Geometry: final body of the model. Coordinates: model frame, mm. A direction names the side the tool comes from. Give positions to 0.01 mm unless a question says otherwise; leave off trailing zeros. Write each loop counter-clockwise with the first axis right and the second up, starting at its lowest first coordinate (ties: lowest second). Pieces come first, ordered by that corner, then holes. Notation, with made-up numbers: M 14,8.25 L 61,8.25 A19 ccw 61,37.25 Z; hole C 78.25,0.25 d10. An arc over 180 degrees is marked long. Answer as a JSON object with one key per item and string values.
from build123d import *

# Parameters (mm, degrees)
F0_R     = 17.5
F1_DEPTH = 5
F2_R     = 15.5
F3_DEPTH = 3
F4_R     = 3.5
F4_R_2   = 1.5
F5_DEPTH = 6
F7_DEPTH = 1
F8_DEPTH = 2


with BuildPart() as f1:
    # F0 (on Top) → F1 (new body)
    with BuildSketch(Plane.XY):
        Circle(F0_R)
    extrude(amount=F1_DEPTH)

    # F2 (on face) → F3 (cut)
    with BuildSketch(Plane.XY.offset(5)):
        Circle(F2_R)
    extrude(amount=-F3_DEPTH, mode=Mode.SUBTRACT)

    # F4 (on face) → F5 (join)
    with BuildSketch(Plane.XY.offset(2)):
        Circle(F4_R)
        Circle(F4_R_2, mode=Mode.SUBTRACT)
    extrude(amount=F5_DEPTH)

    # F6 (on face) → F7 (cut)
    with BuildSketch(Plane(origin=(0, 0, 0), x_dir=(1, 0, 0), z_dir=(0, 0, -1))):
        Polygon((-3.9243327608, 0.1564746204), (-3.3940706843, 1.1028004157), (-3.2668253693, 2.1800742948), (-12.161596097, 3.9515421095), align=None)
        Polygon((1.0638693073, 3.7806155611), (0, 12.7874588824), (-1.0638693073, 3.7806155611), (0, 3.5687371109), align=None)
        Polygon((3.2668253693, 2.1800742948), (3.3940706843, 1.1028004157), (3.9243327608, 0.1564746204), (12.161596097, 3.9515421095), align=None)
        Polygon((3.0828784209, -2.4332555489), (2.0976510431, -2.8871689712), (1.361501722, -3.6839089274), (7.5162797454, -10.3452715508), align=None)
        Polygon((-1.361501722, -3.6839089274), (-2.0976510431, -2.8871689712), (-3.0828784209, -2.4332555489), (-7.5162797454, -10.3452715508), align=None)
    extrude(amount=-F7_DEPTH, mode=Mode.SUBTRACT)

    # F6 (on face) → F8 (cut)
    with BuildSketch(Plane(origin=(0, 0, 0), x_dir=(1, 0, 0), z_dir=(0, 0, -1))):
        with BuildLine():
            Line((7.6763518896, -13.4656459803), (0, -5.1574724983))
            Line((0, -5.1574724983), (-7.6763518896, -13.4656459803))
            ThreePointArc((-7.6763518896, -13.4656459803), (0, -15.5), (7.6763518896, -13.4656459803))
        make_face()
        with BuildLine():
            Line((-10.434467167, -11.4617579341), (-4.9050478272, -1.59374665))
            Line((-4.9050478272, -1.59374665), (-15.1787135444, 3.1395310378))
            ThreePointArc((-15.1787135444, 3.1395310378), (-14.7413760026, -4.7897634128), (-10.434467167, -11.4617579341))
        make_face()
        with BuildLine():
            Line((1.7046089863, 15.4059828704), (3.0314862736, 4.1724828992))
            Line((3.0314862736, 4.1724828992), (14.1252072533, 6.3818900062))
            ThreePointArc((14.1252072533, 6.3818900062), (9.1106714105, 12.5397634128), (1.7046089863, 15.4059828704))
        make_face()
        with BuildLine():
            Line((15.1787135444, 3.1395310378), (4.9050478272, -1.59374665))
            Line((4.9050478272, -1.59374665), (10.434467167, -11.4617579341))
            ThreePointArc((10.434467167, -11.4617579341), (14.1771689891, -6.2656108605), (15.5, 0))
            ThreePointArc((15.5, 0), (15.4194691857, 1.5779638877), (15.1787135444, 3.1395310378))
        make_face()
        with BuildLine():
            Line((-14.1252072533, 6.3818900062), (-3.0314862736, 4.1724828992))
            Line((-3.0314862736, 4.1724828992), (-1.7046089863, 15.4059828704))
            ThreePointArc((-1.7046089863, 15.4059828704), (-9.1106714105, 12.5397634128), (-14.1252072533, 6.3818900062))
        make_face()
    extrude(amount=-F8_DEPTH, mode=Mode.SUBTRACT)


solid = f1.part
1) Cut plane D-D on y = 6.5. Return loops of the section in (x, z).
Geometry check:
{"outline": "M -16.25,0 L -14.07,0 L -14.07,5 L -16.25,5 Z; M -7.65,0 L -5.36,0 L -5.36,1 L -3.96,1 L -3.96,0 L -1.24,0 L -1.24,2 L -7.65,2 Z; M 1.24,0 L 3.96,0 L 3.96,1 L 5.36,1 L 5.36,0 L 7.65,0 L 7.65,2 L 1.24,2 Z; M 14.07,0 L 16.25,0 L 16.25,5 L 14.07,5 Z"}
2) Cut plane B-B on y = -13.5. Return loops of the section in (x, z).
Geometry check:
{"outline": "M -11.14,0 L -7.62,0 L -7.62,5 L -11.14,5 Z; M -1.93,0 L 1.93,0 L 1.93,2 L -1.93,2 Z; M 7.62,0 L 11.14,0 L 11.14,5 L 7.62,5 Z"}
3) Cut plane A-A on z = 3.75. Return loops of the section in (x, y), and give its area (3 significant figures).
Geometry check:
{"outline": "C 0,0 d35; C 0,0 d7; hole C 0,0 d31; hole C 0,0 d3", "area": "239 mm2"}
4) Contact query for a flat-ended pin moving along its axis: P1, Ø5, axis at x = -9.5, y = 6, coming from the +Z side. Output: stop coordinate, or through.
Geometry check:
{"P1": "stops at z = 2"}
5) Cut plane C-C on x = 9. Return loops of the section in (y, z).
Geometry check:
{"outline": "M -15.01,0 L -12.62,0 L -12.62,5 L -15.01,5 Z; M -5.36,0 L -3.32,0 L -3.32,1 L -2.49,1 L -2.49,0 L -0.29,0 L -0.29,2 L -5.36,2 Z; M 8.9,0 L 15.01,0 L 15.01,5 L 12.62,5 L 12.62,2 L 8.9,2 Z"}
6) Set-up query: faces 3 (the flat face through (3.655, -0.636, 0.493)), 4 (the flat face through (10.1, -0.8, 1)). Return all of +Z, -Z, +X, -X, +Y, -Y with unobstructed straight access to the full face (end or side cutting, diameter ignored); none if empty.
Geometry check:
{"face 3": "-Z", "face 4": "+Z, -Z"}
7) Pull-direction query (X, two-part tool) for faces 1 (the flat face through (-7.71, 6.6, 0.99)), 2 (the flat face through (0, -2, 8)); classes: pulls with the +X half, pulls with the -X half, needs draft (parallel to the pull), parting line crosses it, or undercut.
Geometry check:
{"face 1": "undercut", "face 2": "needs draft"}
8) Line query: line 1 (Y direction, x = 0, z = 4.35); line 2 (Y direction, x = 0, z = 5.3); line 3 (X direction, y = -8, z = 0.75). Output: solid intervals per line, ascending. Write a range as from..to.
Geometry check:
{"line 1": "y = -17.5..-15.5, -3.5..-1.5, 1.5..3.5, 15.5..17.5", "line 2": "y = -3.5..-1.5, 1.5..3.5", "line 3": "x = -15.56..-13.28, -2.58..-0.57, 0.57..2.58, 13.28..15.56"}
